Answer from the drawing. Dimensions are ordinates in mm from the lowest x, y and z of the part. A direction names the side the tool comes from. Coordinates: 2 decimals unless noted, no trailing zeros. Write each loop counter-clockwise with the first axis right and the second up, starting at its lowest first coordinate (ties: lowest second). Pieces come first, ordered by that corner, then holes.
(1) Find the intervals of material crossed by probe 1 along X at (y, z) = (16.25, 1.15); probe 2 along Y at (x, z) = (7.25, 1.15) (1 decimal); probe 3 along X at (y, z) = (7.75, 2.5) (1 decimal), in increasing order.
(2) Which of the six approach directions +Z, -Z, +X, -X, +Y, -Y give full straight-line access (tool end or side, diameter ignored) to the marked faces 1 and 2?
(3) Given pin 1 (6.5 mm diameter, centred on x = 8.5, y = 11.5, fed in from -Z), flat-ended and moving along its own axis, determine where the tip first touches the part or whether it passes through.
(4) Section C-C on y = 12.25 is taken. Write down the section's boundary in (x, z) (1 decimal).
(5) The mould has two halves that part along X. Classify the marked faces 3, 4, 5 and 6: +X half, -X half, draft (parallel to the pull), parting line (faces both ways), or undercut.
(6) Section B-B on x = 14 is taken. Write down the section's boundary in (y, z) (1 decimal).
(7) Section A-A on z = 0.4 is taken. Write down the section's boundary in (x, y) (1 decimal).
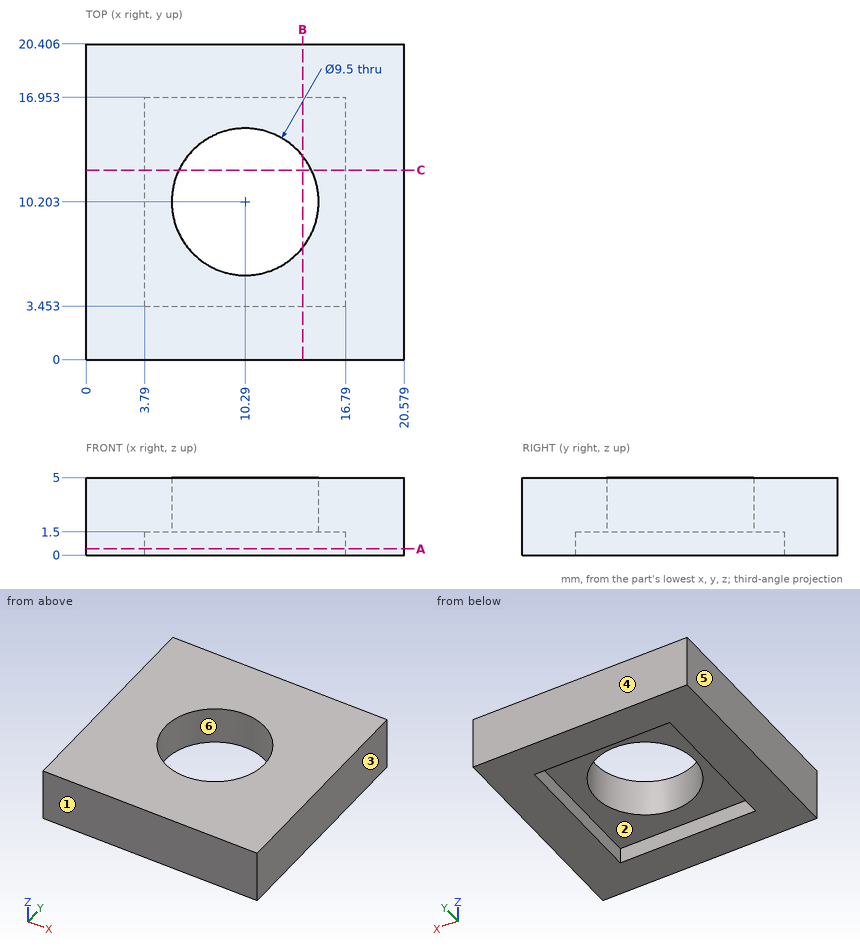
Response:
1. probe 1: x = 0 to 3.79, 16.79 to 20.58
1. probe 2: y = 0 to 3.5, 17 to 20.4
1. probe 3: x = 0 to 6.2, 14.4 to 20.6
2. face 1: +Z, -Z, +X, -X, -Y
2. face 2: -Z
3. pin 1: stops at z = 1.5
4. outline: (0, 0) - (3.8, 0) - (3.8, 1.5) - (6, 1.5) - (6, 5) - (0, 5) - close; (14.6, 1.5) - (16.8, 1.5) - (16.8, 0) - (20.6, 0) - (20.6, 5) - (14.6, 5) - close
5. face 3: +X half
5. face 4: draft
5. face 5: -X half
5. face 6: undercut
6. outline: (0, 0) - (3.5, 0) - (3.5, 1.5) - (7.2, 1.5) - (7.2, 5) - (0, 5) - close; (13.2, 1.5) - (17, 1.5) - (17, 0) - (20.4, 0) - (20.4, 5) - (13.2, 5) - close
7. outline: (0, 0) - (20.6, 0) - (20.6, 20.4) - (0, 20.4) - close; hole (3.8, 3.5) - (16.8, 3.5) - (16.8, 17) - (3.8, 17) - close
